Source: CAD feature listing. Evaluate the final solid. Frame: model axes, mm. Face numbers are marked on the shaded views. A direction names the side the tool comes from. Round coordinates to 2 decimals unless told otherwise and drop trailing zeros. Order: outer loops, then holes, each group sorted by start corner. A loop starts at its lowest first (then second) coordinate and runs counter-clockwise, first axis right, second up. Notation, with made-up numbers: (-8.75, 10.25) -> (11.25, 10.25) arc R11 cw to (11.25, 30.25) -> close; hole circle Ø5 at (56.25, 74). An arc over 180 degrees is marked (long way). Use a Markdown table: item, result. Add a question column.
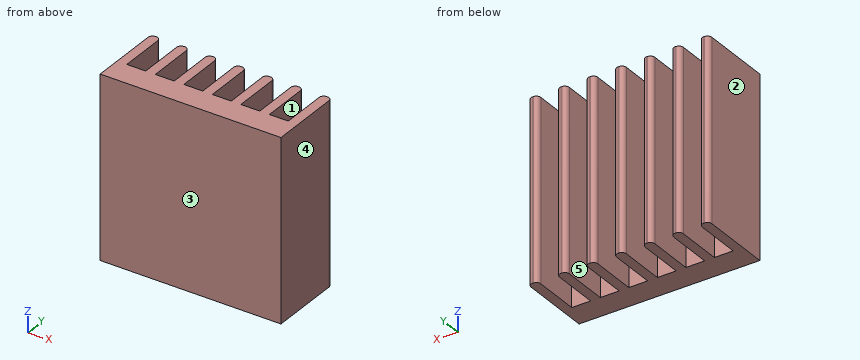
```python
from build123d import *

# Parameters (mm, degrees)
SKETCH1_W           = 14.4
SKETCH1_H           = 14.4
BOSS_EXTRUDE1_DEPTH = 2
SKETCH2_W           = 0.77
SKETCH2_H           = 4
BOSS_EXTRUDE2_DEPTH = 14.4
FILLET1_R           = 0.35


with BuildPart() as part:
    # Sketch1 → Boss-Extrude1 (new body)
    with BuildSketch(Plane(origin=(0, 0, 0), x_dir=(1, 0, 0), z_dir=(0, 1, 0))):
        with Locations((7.2, 7.2)):
            Rectangle(SKETCH1_W, SKETCH1_H)
    extrude(amount=-BOSS_EXTRUDE1_DEPTH)

    # Sketch2 → Boss-Extrude2 (add)
    with BuildSketch(Plane.XY):
        with Locations((2.656666667, 2)):
            Rectangle(SKETCH2_W, SKETCH2_H)
        with Locations((0.385, 2)):
            Rectangle(SKETCH2_W, SKETCH2_H)
        with Locations((4.928333333, 2)):
            Rectangle(SKETCH2_W, SKETCH2_H)
        with Locations((7.2, 2)):
            Rectangle(SKETCH2_W, SKETCH2_H)
        with Locations((9.471666667, 2)):
            Rectangle(SKETCH2_W, SKETCH2_H)
        with Locations((11.743333333, 2)):
            Rectangle(SKETCH2_W, SKETCH2_H)
        with Locations((14.015, 2)):
            Rectangle(SKETCH2_W, SKETCH2_H)
    extrude(amount=-BOSS_EXTRUDE2_DEPTH)

    # Fillet1
    fillet1_edges = [part.edges().sort_by_distance(p)[0] for p in [
        (0.77, 4, -7.2),
        (0, 4, -7.2),
        (3.041666667, 4, -7.2),
        (2.271666667, 4, -7.2),
        (5.313333333, 4, -7.2),
        (4.543333333, 4, -7.2),
        (7.585, 4, -7.2),
        (6.815, 4, -7.2),
        (9.856666667, 4, -7.2),
        (9.086666667, 4, -7.2),
        (12.128333333, 4, -7.2),
        (11.358333333, 4, -7.2),
        (14.4, 4, -7.2),
        (13.63, 4, -7.2),
    ]]
    fillet(fillet1_edges, radius=FILLET1_R)


solid = part.part
```
1) Line query: probe 1 along Y at (x, z) = (10, -11); probe 2 along Y at (x, z) = (2.5, -6.5). Output: solid intervals per line, ascending. Write a range as from..to.
2) First-contact query: pin 1 Ø0.8 at (x, z) = (8.5, -8) entering from +Y. Flat tip, straight axial feed; report the tip coordinate or a pass-through.
3) Reachability of the marked faces 4 and 5 from +Z, -Z, +X, -X, +Y, -Y: full face, straight path, thin tool, end or side. Return the list, or none.
4) Draft query along X for the marked faces 1, 2 and 3. Return one class per face: pulls with the +X half, pulls with the -X half, needs draft (parallel to the pull), parting line crosses it, or undercut.
5) Section A-A on y = 0.35. Output: boundary loops of the cut face in (x, z) (3 decimals), then the cut area to 3 significant figures.
6) Section B-B on x = 10.5. Output: boundary loops of the cut face in (y, z), then the cut area to 3 significant figures.
Conclusion:
| question | item | result |
|---|---|---|
| 1 | probe 1 | y = -2..0 |
| 1 | probe 2 | y = -2..3.98 |
| 2 | pin 1 | stops at y = 0 |
| 3 | face 4 | +Z, -Z, +X, +Y, -Y |
| 3 | face 5 | +Z, -Z, +Y |
| 4 | face 1 | undercut |
| 4 | face 2 | pulls with the -X half |
| 4 | face 3 | needs draft |
| 5 | outline | (0, -14.4) -> (0.77, -14.4) -> (0.77, 0) -> (0, 0) -> close; (2.272, -14.4) -> (3.042, -14.4) -> (3.042, 0) -> (2.272, 0) -> close; (4.543, -14.4) -> (5.313, -14.4) -> (5.313, 0) -> (4.543, 0) -> close; (6.815, -14.4) -> (7.585, -14.4) -> (7.585, 0) -> (6.815, 0) -> close; (9.087, -14.4) -> (9.857, -14.4) -> (9.857, 0) -> (9.087, 0) -> close; (11.358, -14.4) -> (12.128, -14.4) -> (12.128, 0) -> (11.358, 0) -> close; (13.63, -14.4) -> (14.4, -14.4) -> (14.4, 0) -> (13.63, 0) -> close |
| 5 | area | 77.6 mm^2 |
| 6 | outline | (-2, -14.4) -> (0, -14.4) -> (0, 0) -> (-2, 0) -> close |
| 6 | area | 28.8 mm^2 |
